Autodesk Inventor part; units mm, degrees
ref_plane "YZ Plane" through (0, 0, 0) normal (1, 0, 0) x (0, 1, 0)
ref_plane "XZ Plane" through (0, 0, 0) normal (0, 1, 0) x (-1, 0, 0)
ref_plane "XY Plane" through (0, 0, 0) normal (0, 0, 1) x (1, 0, 0)
sketch "Sketch1" plane through (0, 0, 0) normal (0, 1, 0) x (-1, 0, 0)
  point P0 (0, 0)
sketch "Sketch2" plane through (0, 0, 0) normal (0, 1, 0) x (-1, 0, 0)
  line L0 (0, 0) -> (-50, 0)
  line L1 (-50, 0) -> (-50, -120)
  line L2 (-50, -120) -> (0, -120)
  line L3 (0, -120) -> (0, 0)
  line L4 (-20, -23.5) -> (-43, -23.5)
  line L5 (-43, -23.5) -> (-43, -26.75)
  line L6 (-43, -26.75) -> (-45, -26.75)
  line L7 (-45, -26.75) -> (-45, -33.25)
  line L8 (-45, -33.25) -> (-43, -33.25)
  line L9 (-43, -33.25) -> (-43, -36.5)
  line L10 (-43, -36.5) -> (-20, -36.5)
  line L11 (-20, -36.5) -> (-20, -23.5)
  line L12 (-20, -43.5) -> (-43, -43.5)
  line L13 (-43, -43.5) -> (-43, -46.75)
  line L14 (-43, -46.75) -> (-45, -46.75)
  line L15 (-45, -46.75) -> (-45, -53.25)
  line L16 (-45, -53.25) -> (-43, -53.25)
  line L17 (-43, -53.25) -> (-43, -56.5)
  line L18 (-43, -56.5) -> (-20, -56.5)
  line L19 (-20, -56.5) -> (-20, -43.5)
  line L20 (-20, -63.5) -> (-43, -63.5)
  line L21 (-43, -63.5) -> (-43, -66.75)
  line L22 (-43, -66.75) -> (-45, -66.75)
  line L23 (-45, -66.75) -> (-45, -73.25)
  line L24 (-45, -73.25) -> (-43, -73.25)
  line L25 (-43, -73.25) -> (-43, -76.5)
  line L26 (-43, -76.5) -> (-20, -76.5)
  line L27 (-20, -76.5) -> (-20, -63.5)
  circle A0 centre (-17.5, -50) radius 1
  circle A1 centre (-17.5, -70) radius 1
  circle A2 centre (-17.5, -30) radius 1
  circle A3 centre (-47.4974, -30) radius 1
  circle A4 centre (-47.5, -50) radius 1
  circle A5 centre (-47.5, -70) radius 1
  dimension "d0" = 50
  dimension "d1" = 120
  dimension "d4" = 23
  dimension "d5" = 3.25
  dimension "d6" = 2
  dimension "d7" = 6.5
  dimension "d8" = 2
  dimension "d9" = 3.25
  dimension "d10" = 23
  dimension "d12" = 23
  dimension "d13" = 3.25
  dimension "d14" = 2
  dimension "d15" = 6.5
  dimension "d16" = 2
  dimension "d17" = 3.25
  dimension "d18" = 23
  dimension "d20" = 23
  dimension "d21" = 3.25
  dimension "d22" = 2
  dimension "d23" = 6.5
  dimension "d24" = 3.25
  dimension "d25" = 23
  dimension "d29" = 2
  dimension "d30" = 2
  dimension "d31" = 2
  dimension "d32" = 2
  dimension "d35" = 2
  dimension "d36" = 2
extrude "Extrusion1" add sketch "Sketch2" along normal blind 3
properties part number "Part1_FInal"
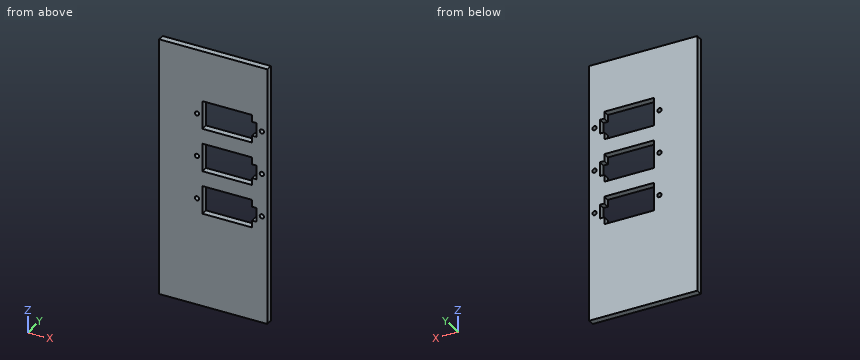
Could you check a few things on this model? Use its own coordinates, in mm. Round coordinates to 2 decimals unless told otherwise and drop trailing zeros. Loops run counter-clockwise (first coordinate to the right, second up) from the corner with the lowest first, then second, coordinate; pieces in that order, holes last. Notation, with made-up numbers: (83.5, 57.5) - (95.5, 57.5) arc R17 ccw to (95.5, 69.5) - close; hole circle Ø5 at (20, -19). An arc over 180 degrees is marked (long way). Write item = value, one per line.
1) I'm going to push a flat-ended pin straight in: P1, Ø6, axis at x = 42.5, z = -25.5, coming from the -Y side. Where does the tip first touch, or does it pass through?
Computed:
P1 = 0
2) Imagine slicing it at A-A (x = 38.5). Please give me the cut outline in (y, z), and give its area (3 significant figures).
Computed:
outline = (0, -120) - (3, -120) - (3, -76.5) - (0, -76.5) - close; (0, -63.5) - (3, -63.5) - (3, -56.5) - (0, -56.5) - close; (0, -43.5) - (3, -43.5) - (3, -36.5) - (0, -36.5) - close; (0, -23.5) - (3, -23.5) - (3, 0) - (0, 0) - close
area = 243 mm2
3) I need wall thicknesses on line 1 along Z through (x, y) = (17.5, 1.3); line 2 along Z through (x, y) = (36, 1.3); line 3 along X through (y, z) = (1.1, -70). Which ranges of each line are inside material? Lowest first, please. Write a range as from..to.
Computed:
line_1 = -120..-71, -69..-51, -49..-31, -29..0
line_2 = -120..-76.5, -63.5..-56.5, -43.5..-36.5, -23.5..0
line_3 = 0..16.5, 18.5..20, 45..46.5, 48.5..50
4) Imagine slicing it at B-B (y = 1.3). Give the number of separate pieces and of enclosed holes in the cut face, and give its area (3 significant figures).
Computed:
separate_pieces = 1
enclosed_holes = 9
area = 5,050 mm2
